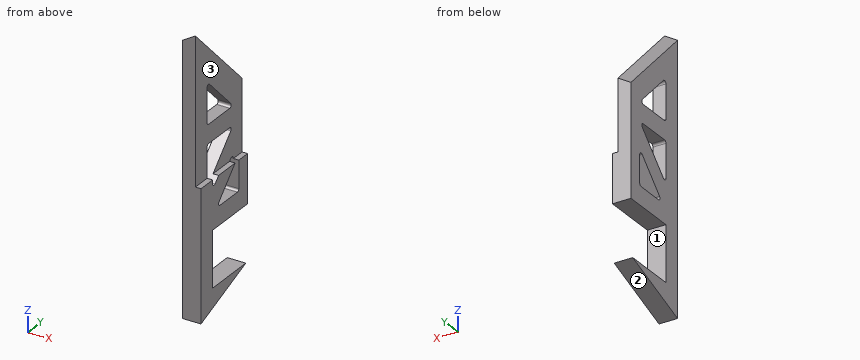
from build123d import *

# Parameters (mm, degrees)
BOSS_EXTRUDE1_DEPTH    = 12.7
CUT_EXTRUDE1_START     = -62.002468855
CUT_EXTRUDE1_OUTLINE_W = 16
CUT_EXTRUDE1_OUTLINE_H = 80
CUT_EXTRUDE1_DEPTH     = 4.960197509
CUT_EXTRUDE2_START     = 12.7
CUT_EXTRUDE2_DEPTH     = 3.81
CUT_EXTRUDE3_REACH     = 110.694
FILLET1_R              = 1.5875


# Read off the part's stored shape, not the designer's step: Cut-Extrude1
with BuildPart() as part:
    # Sketch1 → Boss-Extrude1 (new body)
    with BuildSketch(Plane(origin=(0, 0, 0), x_dir=(0, 0, -1), z_dir=(1, 0, 0))):
        Polygon((-44.45, 50.8), (-95.25, 0), (95.25, 0), (77.47, 48.850148518), (77.47, 12.7), (39.37, 12.7), (39.37, 50.8), align=None)
    extrude(amount=BOSS_EXTRUDE1_DEPTH)

    # Cut-Extrude1 outline → Cut-Extrude1 (cut)
    with BuildSketch(Plane(origin=(0, 0, 0), x_dir=(0.920574617898324, 0.27617238536949745, 0.27617238536949446), z_dir=(0.39056673294247013, -0.6509445549041233, -0.6509445549041163)).offset(CUT_EXTRUDE1_START)):
        with Locations((31, 29)):
            Rectangle(CUT_EXTRUDE1_OUTLINE_W, CUT_EXTRUDE1_OUTLINE_H)
    extrude(amount=CUT_EXTRUDE1_DEPTH, mode=Mode.SUBTRACT)

    # Sketch1<4> → Cut-Extrude2 (cut)
    with BuildSketch(Plane(origin=(0, 0, 0), x_dir=(0, 0, -1), z_dir=(1, 0, 0)).offset(CUT_EXTRUDE2_START)):
        Polygon((-44.45, 50.8), (-95.25, 0), (6.35, 0), (6.35, 50.8), align=None)
    extrude(amount=-CUT_EXTRUDE2_DEPTH, mode=Mode.SUBTRACT)

    # Sketch3 → Cut-Extrude3 (cut, up to next)
    with BuildSketch(Plane.ZY, mode=Mode.PRIVATE) as cut_extrude3_sk1:
        Polygon((56.969487758, 12.7), (28.394487758, 41.275), (28.394487758, 12.7), align=None)
    cut_extrude3_tool1 = extrude(cut_extrude3_sk1.sketch, amount=-CUT_EXTRUDE3_REACH, mode=Mode.PRIVATE) & part.part
    # Sketch3 → Cut-Extrude3 (cut, up to next)
    with BuildSketch(Plane.ZY, mode=Mode.PRIVATE) as cut_extrude3_sk2:
        Polygon((15.694487758, 41.275), (15.694487758, 12.7), (-12.880512242, 12.7), align=None)
    cut_extrude3_tool2 = extrude(cut_extrude3_sk2.sketch, amount=-CUT_EXTRUDE3_REACH, mode=Mode.PRIVATE) & part.part
    # Sketch3 → Cut-Extrude3 (cut, up to next)
    with BuildSketch(Plane.ZY, mode=Mode.PRIVATE) as cut_extrude3_sk3:
        Polygon((-2.266024484, 41.275), (-26.67, 16.871024484), (-26.67, 41.275), align=None)
    cut_extrude3_tool3 = extrude(cut_extrude3_sk3.sketch, amount=-CUT_EXTRUDE3_REACH, mode=Mode.PRIVATE) & part.part
    add(cut_extrude3_tool1.solids().sort_by_distance((0, 22.225, 37.919488))[0], mode=Mode.SUBTRACT)
    add(cut_extrude3_tool2.solids().sort_by_distance((0, 22.225, 6.169488))[0], mode=Mode.SUBTRACT)
    add(cut_extrude3_tool3.solids().sort_by_distance((0, 33.140341, -18.535341))[0], mode=Mode.SUBTRACT)

    # Fillet1
    fillet1_edges = [part.edges().sort_by_distance(p)[0] for p in [
        (4.445, 12.7, 56.969487758),
        (4.445, 12.7, 28.394487758),
        (4.445, 41.275, 28.394487758),
        (6.35, 41.275, -26.67),
        (4.445, 41.275, -2.266024484),
        (6.35, 16.871024484, -26.67),
        (4.445, 41.275, 15.694487758),
        (6.35, 12.7, -12.880512242),
        (4.445, 12.7, 15.694487758),
    ]]
    fillet(fillet1_edges, radius=FILLET1_R)


solid = part.part
Design review of the part built by this model. Coordinates are the model's own, in mm. Face numbers are marked on the shaded views. A direction names the side the tool comes from. Give positions to 0.01 mm unless a question says otherwise; leave off trailing zeros. Write each loop counter-clockwise with the first axis right and the second up, starting at its lowest first coordinate (ties: lowest second). Pieces come first, ordered by that corner, then holes. Notation, with made-up numbers: M -34,-21.5 L -23,-21.5 A12 cw -23,-7.5 Z; hole C 65.25,15.5 d10. An arc over 180 degrees is marked long. Answer as a JSON object with one key per item and string values. Group by question number.
1) Clearance check with flat-ended pins moving along their axes: pin 1 Ø5 at (x, z) = (2.5, 63.5) entering from -Y; pin 2 Ø1.1 at (x, y) = (10, 31.5) entering from +Z; pin 3 Ø6 at (x, y) = (11.5, 29.5) entering from -Z; pin 4 Ø1.5 at (x, y) = (8.5, 15.5) entering from -Z. State where each tip first meets the part, or that it passes through.
2) We need section D-D (y = 17). Give the boundary of the cut face in (x, z).
3) We need section A-A (x = 5.5). Count the separate pieces of the cut face and the enclosed holes in it, and give its area (3 significant figures).
4) Tool access review of the marked faces 1, 2 and 3: name each direction out of +Z, -Z, +X, -X, +Y, -Y from which nothing blocks a thin tool from reaching the whole face with its end or side.
5) We need section B-B (z = 46). Give the boundary of the cut face in (x, y).
6) For line 1 along Z through (x, y) = (3, 41); line 2 along Y through (x, z) = (2.75, -25) (3 decimals); line 3 along Z through (x, y) = (3, 28.5), list the stretches that pass through material, from the lowest coordinate up.
7) We need section C-C (y = 44). Give the boundary of the cut face in (x, z).
Answer key:
{
 "1": {"pin 1": "stops at y = 0", "pin 2": "stops at z = -6.35", "pin 3": "stops at z = -85.6", "pin 4": "stops at z = -89.88"},
 "2": {"outline": "M 0,-89.06 L 12.7,-89.06 L 12.7,-77.47 L 0,-77.47 Z; M 0,-39.37 L 12.7,-39.37 L 12.7,-8.58 L 0,-8.58 Z; M 0,15.69 L 8.89,15.69 L 8.89,28.39 L 0,28.39 Z; M 0,52.67 L 8.89,52.67 L 8.89,75.96 L 0,70.63 Z"},
 "3": {"separate pieces": "1", "enclosed holes": "3", "area": "5,150 mm²"},
 "4": {"face 1": "+X, -X, +Y", "face 2": "-Z, +X, -X, +Y", "face 3": "+Z, +X, +Y, -Y"},
 "5": {"outline": "M 0,0 L 8.89,0 L 8.89,12.7 L 0,12.7 Z; M 0,23.67 L 8.89,23.67 L 8.89,46.96 L 0,41.63 Z"},
 "6": {"line 1": "z = -80.33 to -77.47, -39.37 to -25.98, -5.21 to 48.43", "line 2": "y = 0 to 19.118, 41.275 to 50.8", "line 3": "z = -84.88 to -77.47, -39.37 to -26.67, -15.04 to 2.92, 15.69 to 28.39, 41.17 to 60.93"},
 "7": {"outline": "M 0,-79.24 L 12.7,-79.24 L 12.7,-77.47 L 0,-77.47 Z; M 0,-39.37 L 12.7,-39.37 L 12.7,-6.35 L 8.89,-6.35 L 8.89,48.96 L 0,43.63 Z"}
}
